The figure shows three views and two pictorial views of one solid part (mm, origin at its lowest corner). Answer the questions. A direction names the side the tool comes from. Give positions to 0.01 mm unless a question says otherwise; leave off trailing zeros. Order: outer loops, then holes, each group sorted by start corner. A loop starts at its lowest first (then second) coordinate and runs counter-clockwise, first axis right, second up. Notation, with made-up numbers: (45, -24.5) -> (67, -24.5) arc R8 cw to (67, -14.5) -> close; hole circle Ø4 at (72, 6.5). An arc over 180 degrees is marked (long way). One line per item, written item: value. Start each with the question number.
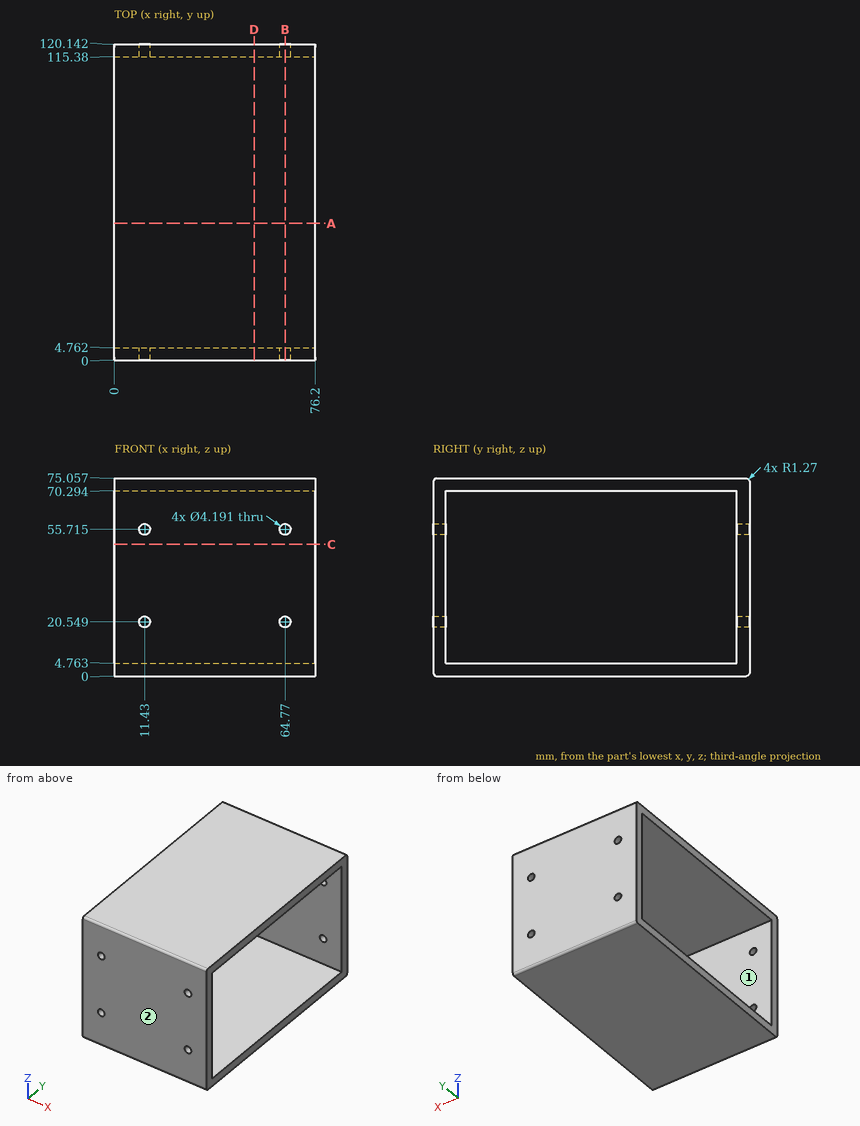
Item 1: Find section C-C on z = 50. Write down the section's boundary in (x, y).
Item 2: Find section B-B on x = 64.77. Write down the section's boundary in (y, z) (1 decimal), then the cut area to 3 significant figures.
Item 3: Find the intervals of material crossed by line 1 (Z direction, x = 62, y = 59.5) (1 decimal); line 2 (Y direction, x = 26, z = 21.5); line 3 (Z direction, x = 64.77, y = 116.4) (1 decimal), in increasing order. Write a range as from..to.
Item 4: A tool of negligible diameter and unlimited length cuts with its end or side. For the marked faces 1 and 2, from which of +Z, -Z, +X, -X, +Y, -Y can it reach the whole face along a straight path? Write none if from no direction.
Item 5: Find section A-A on y = 52. Write down the section's boundary in (x, z) (1 decimal).
Item 6: Find section D-D on x = 53. Write down the section's boundary in (y, z) (1 decimal).
Checks:
1. outline: (0, 0) -> (76.2, 0) -> (76.2, 4.76) -> (0, 4.76) -> close; (0, 115.38) -> (76.2, 115.38) -> (76.2, 120.14) -> (0, 120.14) -> close
2. outline: (0, 1.3) arc R1.3 ccw to (1.3, 0) -> (118.9, 0) arc R1.3 ccw to (120.1, 1.3) -> (120.1, 18.5) -> (115.4, 18.5) -> (115.4, 4.8) -> (4.8, 4.8) -> (4.8, 18.5) -> (0, 18.5) -> close; (0, 22.6) -> (4.8, 22.6) -> (4.8, 53.6) -> (0, 53.6) -> close; (0, 57.8) -> (4.8, 57.8) -> (4.8, 70.3) -> (115.4, 70.3) -> (115.4, 57.8) -> (120.1, 57.8) -> (120.1, 73.8) arc R1.3 ccw to (118.9, 75.1) -> (1.3, 75.1) arc R1.3 ccw to (0, 73.8) -> close; (115.4, 22.6) -> (120.1, 22.6) -> (120.1, 53.6) -> (115.4, 53.6) -> close
2. area: 1,690 mm2
3. line 1: 0..4.8, 70.3..75.1
3. line 2: 0..4.76, 115.38..120.14
3. line 3: 0..18.5, 22.6..53.6, 57.8..75.1
4. face 1: +X, -X
4. face 2: +Z, -Z, +X, -X, -Y
5. outline: (0, 0) -> (76.2, 0) -> (76.2, 4.8) -> (0, 4.8) -> close; (0, 70.3) -> (76.2, 70.3) -> (76.2, 75.1) -> (0, 75.1) -> close
6. outline: (0, 1.3) arc R1.3 ccw to (1.3, 0) -> (118.9, 0) arc R1.3 ccw to (120.1, 1.3) -> (120.1, 73.8) arc R1.3 ccw to (118.9, 75.1) -> (1.3, 75.1) arc R1.3 ccw to (0, 73.8) -> close; hole (4.8, 4.8) -> (115.4, 4.8) -> (115.4, 70.3) -> (4.8, 70.3) -> close
